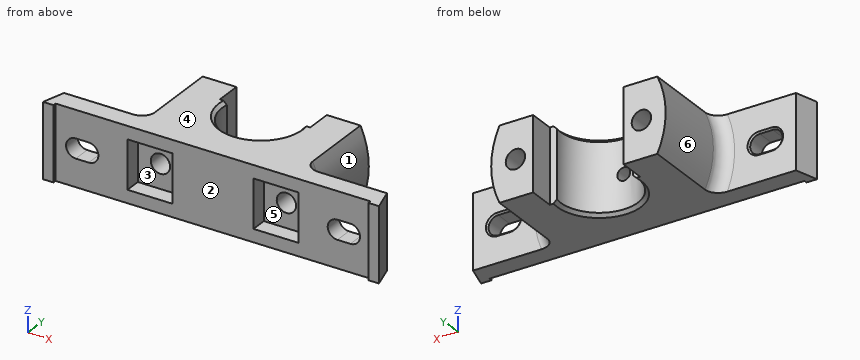
```python
from build123d import *

# Parameters (mm, degrees)
BOSS_EXTRUDE1_DEPTH     = 23
CUT_EXTRUDE5_DEPTH      = 54
FILLET1_R               = 8
CHAMFER1_SIZE           = 2
CUT_EXTRUDE2_DEPTH      = 117.82893492196186
CUT_EXTRUDE2_DEPTH_BACK = 117.82893492196186
SKETCH4_W               = 195
SKETCH4_H               = 2
CUT_EXTRUDE6_DEPTH      = 120.41942905658195
SKETCH5_W               = 28.000000000000004
SKETCH5_H               = 30
SKETCH5_R               = 6.000000000000002
CUT_EXTRUDE3_DEPTH      = 10
SKETCH5_2_R             = 6.000000000000002
CUT_EXTRUDE7_DEPTH      = 126.30363138632497
CHAMFER2_SIZE           = 1
SKETCH9_R               = 4
CUT_EXTRUDE8_DEPTH      = 36


with BuildPart() as part:
    # Sketch1 → Boss-Extrude1 (new, symmetric)
    with BuildSketch(Plane.XY):
        with BuildLine():
            Line((-104, -48), (104, -48))
            Line((104, -48), (99.98556459937663, -34))
            Line((99.98556459937663, -34), (54.00000000000001, -34.00000000000001))
            Line((54.00000000000001, -34.00000000000001), (54.00000000000001, 20))
            Line((54.00000000000001, 20), (28.000000000000004, 20))
            Line((28.000000000000004, 20), (28, 4))
            Line((28, 4), (23.664319132398468, 4))
            ThreePointArc((23.664319132398468, 4), (1.47e-15, -24.000000000000004), (-23.664319132398465, 4))
            Line((-23.664319132398465, 4), (-28, 4))
            Line((-28, 4), (-28, 20))
            Line((-28, 20), (-54.00000000000001, 20))
            Line((-54.00000000000001, 20), (-54.00000000000001, -34.00000000000001))
            Line((-54.00000000000001, -34.00000000000001), (-99.98556459937662, -33.99999999999999))
            Line((-99.98556459937662, -33.99999999999999), (-104, -48))
        make_face()
    extrude(amount=BOSS_EXTRUDE1_DEPTH, both=True)

    # Sketch7 → Cut-Extrude5 (cut)
    with BuildSketch(Plane(origin=(0, 20, 0), x_dir=(1, 2.9e-16, 0), z_dir=(-2.9e-16, 1, 0))):
        with BuildLine():
            Line((-54.00000000000001, 23), (-54.00000000000001, 4.0501e-13))
            ThreePointArc((-54.000000000000014, 4.0856e-13), (-52.69855043578576, 11.784005344828431), (-48.856934001224445, 23))
            Line((-48.85693400122444, 23), (-54.00000000000001, 23))
        make_face()
        with BuildLine():
            Line((-54.00000000000001, 4.0501e-13), (-54.00000000000001, -23))
            Line((-54.00000000000001, -23), (-48.85693400122444, -23))
            ThreePointArc((-48.856934001224445, -23.000000000000004), (-52.69855043578586, -11.784005344828039), (-54.000000000000014, 4.0856e-13))
        make_face()
        with BuildLine():
            ThreePointArc((48.85693400122443, 23.000000000000004), (52.69855043578579, 11.784005344828252), (54, 3.286e-14))
            Line((54.00000000000001, 3.553e-14), (54.00000000000001, 23))
            Line((54.00000000000001, 23), (48.856934001224424, 23))
        make_face()
        with BuildLine():
            Line((48.856934001224424, -23), (54.00000000000001, -23))
            Line((54.00000000000001, -23), (54.00000000000001, 3.553e-14))
            ThreePointArc((54, 3.286e-14), (52.698550435785805, -11.784005344828213), (48.85693400122443, -23))
        make_face()
    extrude(amount=-CUT_EXTRUDE5_DEPTH, mode=Mode.SUBTRACT)

    # Fillet1
    fillet1_edges = [part.edges().sort_by_distance(p)[0] for p in [
        (-54.000000000000014, -34.000000000000014, -4.4e-16),
        (54.00000000000001, -33.999999999999986, 4.44e-15),
    ]]
    fillet(fillet1_edges, radius=FILLET1_R)

    # Chamfer1
    chamfer1_edges = [part.edges().sort_by_distance(p)[0] for p in [
        (-4.44e-15, -24.000000000000007, -23),
        (-4.44e-15, -24.000000000000007, 23),
    ]]
    chamfer(chamfer1_edges, length=CHAMFER1_SIZE)

    # Sketch4 → Cut-Extrude2 (cut, two sides: drawn at the far end of the back side and taken through both)
    with BuildSketch(Plane.XY.offset(-CUT_EXTRUDE2_DEPTH_BACK)):
        with Locations((0, -47)):
            Rectangle(SKETCH4_W, SKETCH4_H)
    extrude(amount=CUT_EXTRUDE2_DEPTH + CUT_EXTRUDE2_DEPTH_BACK, mode=Mode.SUBTRACT)

    # Sketch8 → Cut-Extrude6 (cut, through all)
    with BuildSketch(Plane(origin=(-1.026e-14, -34.00000000000002, 0), x_dir=(1, -3e-16, 0), z_dir=(3e-16, 1, 0))):
        with BuildLine():
            Line((-85, 6), (-77, 6))
            ThreePointArc((-77, 6), (-71, 0), (-77, -6))
            Line((-77, -6), (-85, -6))
            ThreePointArc((-85, -6), (-91, 7.3e-16), (-85, 6))
        make_face()
    cut_extrude6 = extrude(amount=-CUT_EXTRUDE6_DEPTH, mode=Mode.SUBTRACT)

    # Sketch5 → Cut-Extrude3 (cut)
    with BuildSketch(Plane.XZ.offset(46)):
        with Locations((-39.00000000000001, -1.78e-15)):
            Rectangle(SKETCH5_W, SKETCH5_H)
        with Locations(Location((-38.99999999999999, -3.47e-15, 0), (0, 0, 270))):
            Circle(SKETCH5_R, mode=Mode.SUBTRACT)
    cut_extrude3 = extrude(amount=-CUT_EXTRUDE3_DEPTH, mode=Mode.SUBTRACT)

    # Sketch5<2> → Cut-Extrude7 (cut, through all)
    with BuildSketch(Plane.XZ.offset(46)):
        with Locations(Location((-38.99999999999999, -3.47e-15, 0), (0, 0, 270))):
            Circle(SKETCH5_2_R)
    cut_extrude7 = extrude(amount=-CUT_EXTRUDE7_DEPTH, mode=Mode.SUBTRACT)

    # Mirror5: Cut-Extrude6, Cut-Extrude3, Cut-Extrude7 across plane
    add(cut_extrude6.mirror(Plane(origin=(0, 0, 0), x_dir=(0, 0, 1), z_dir=(1, 0, 0))), mode=Mode.SUBTRACT)
    add(cut_extrude3.mirror(Plane(origin=(0, 0, 0), x_dir=(0, 0, 1), z_dir=(1, 0, 0))), mode=Mode.SUBTRACT)
    add(cut_extrude7.mirror(Plane(origin=(0, 0, 0), x_dir=(0, 0, 1), z_dir=(1, 0, 0))), mode=Mode.SUBTRACT)

    # Chamfer2
    chamfer2_edges = [part.edges().sort_by_distance(p)[0] for p in [
        (-91.00000000000001, -33.99999999999999, 3.7e-16),
        (-81.00000000000001, -34, 6),
        (-71.00000000000001, -34, -3.7e-16),
        (-81.00000000000001, -34, -6),
        (91, -33.99999999999999, 3.7e-16),
        (81, -34, 6),
        (71, -34, -3.7e-16),
        (81, -34, -6),
    ]]
    chamfer(chamfer2_edges, length=CHAMFER2_SIZE)

    # Sketch9 → Cut-Extrude8 (cut)
    with BuildSketch(Plane(origin=(0, 0, 0), x_dir=(1, 0, 0), z_dir=(0, 1, 0))):
        with Locations(Location((0, 0, 0), (0, 0, 270))):
            Circle(SKETCH9_R)
    extrude(amount=-CUT_EXTRUDE8_DEPTH, mode=Mode.SUBTRACT)


solid = part.part
```
Check sheet for the modelled part. Datum: model origin and axes. Units: mm. Face numbers are marked on the shaded views. A direction names the side the tool comes from. Round coordinates to 2 decimals unless told otherwise and drop trailing zeros. Order: outer loops, then holes, each group sorted by start corner. A loop starts at its lowest first (then second) coordinate and runs counter-clockwise, first axis right, second up. Notation, with made-up numbers: M 4,35.25 L 9,35.25 A6 cw 9,43.25 Z; hole C 0.25,52 d2. An arc over 180 degrees is marked long. Answer in a Markdown table with one row per item.
(1) Draft check along X on the marked faces 4, 5 and 6. Enter one of: +X half, -X half, draft (parallel to the pull), parting line (faces both ways), or undercut.
Findings:
| item | result |
|---|---|
| face 4 | draft |
| face 5 | undercut |
| face 6 | -X half |
(2) Section check D-D on y = -29. Record the boundary of the cut face in (x, z), plus the area to 3 significant figures.
Findings:
| item | result |
|---|---|
| outline | M -49.5,-23 L 49.5,-23 A54.58 ccw 49.5,23 L -49.5,23 A54.58 ccw Z; hole C -39,0 d12; hole C 0,0 d8; hole C 39,0 d12 |
| area | 4,590 mm^2 |
(3) Set-up check for the marked faces 1, 2 and 3: record each of +Z, -Z, +X, -X, +Y, -Y from which the full face is reachable in a straight line by a thin tool's end or side.
Findings:
| item | result |
|---|---|
| face 1 | +X, +Y |
| face 2 | +Z, -Z, -Y |
| face 3 | -Y |
(4) Gauge pin test, flat ends, axial feed: pin 1 (8 mm diameter, centred on x = -68.5, z = -7, fed in from -Y); pin 2 (3 mm diameter, centred on y = -14.5, z = -5, fed in from +X); pin 3 (5 mm diameter, centred on y = -24.5, z = 17.5, fed in from -X). Record the tip position at first contact, or that the pin passes through.
Findings:
| item | result |
|---|---|
| pin 1 | stops at y = -46 |
| pin 2 | stops at x = 53.89 |
| pin 3 | stops at x = -51.87 |
(5) Material ranges on line 1 along X through (y, z) = (-4, 0); line 2 along X through (y, z) = (-1, 0); line 3 along Z through (x, y) = (39, -6), recorded low to high. Write a range as from..to.
Findings:
| item | result |
|---|---|
| line 1 | x = -54..-45, -33..-23.66, 23.66..33, 45..54 |
| line 2 | x = -54..-45, -33..-23.98, 23.98..33, 45..54 |
| line 3 | z = -23..-6, 6..23 |
(6) Section check A-A on x = -82. Record the boundary of the cut face in (y, z).
Findings:
| item | result |
|---|---|
| outline | M -46,-23 L -34,-23 L -34,-7 L -35,-6 L -46,-6 Z; M -46,6 L -35,6 L -34,7 L -34,23 L -46,23 Z |
(7) Section check B-B on y = -38. Record the boundary of the cut face in (x, z), plus the area to 3 significant figures.
Findings:
| item | result |
|---|---|
| outline | M -101.13,-23 L 101.13,-23 L 101.13,23 L -101.13,23 Z; hole M -85,-6 L -77,-6 A6 ccw -77,6 L -85,6 A6 ccw Z; hole M -53,-15 L -25,-15 L -25,15 L -53,15 Z; hole M 25,-15 L 53,-15 L 53,15 L 25,15 Z; hole M 77,-6 L 85,-6 A6 ccw 85,6 L 77,6 A6 ccw Z |
| area | 7,210 mm^2 |
(8) Section check C-C on x = -39. Record the boundary of the cut face in (y, z).
Findings:
| item | result |
|---|---|
| outline | M -46,-23 L 20,-23 L 20,-6 L -36,-6 L -36,-15 L -46,-15 Z; M -46,15 L -36,15 L -36,6 L 20,6 L 20,23 L -46,23 Z |
